CAD build for the part. Positions are in the model's coordinates, mm. Give positions to 0.01 mm unless a question says otherwise; leave off trailing zeros. Order: outer loops, then holes, each group sorted by start corner. A loop starts at its lowest first (then second) coordinate and runs counter-clockwise, first axis right, second up.
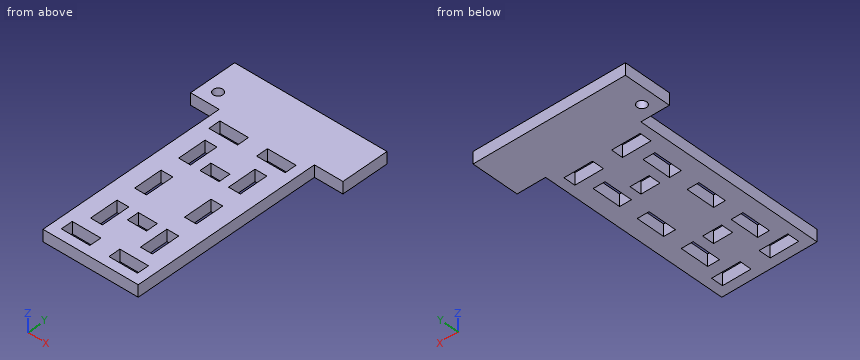
```python
from build123d import *

# Parameters (mm, degrees)
MODEL_R             = 5
MODEL_W             = 12.4
MODEL_H             = 30
MODEL_W_2           = 20
MODEL_H_2           = 12.4
MODEL_W_3           = 30
BOSS_EXTRUDE1_DEPTH = 12.4


with BuildPart() as part:
    # Model → Boss-Extrude1 (new body)
    with BuildSketch(Plane.XY):
        Polygon((50, 200), (80, 200), (80, 250), (-80, 250), (-80, 200), (-50, 200), (-50, 0), (50, 0), align=None)
        with Locations(Location((-65, 215, 0), (0, 0, 180))):
            Circle(MODEL_R, mode=Mode.SUBTRACT)
        with Locations((-26.2, 150)):
            Rectangle(MODEL_W, MODEL_H, mode=Mode.SUBTRACT)
        with Locations((-26.2, 100)):
            Rectangle(MODEL_W, MODEL_H, mode=Mode.SUBTRACT)
        with Locations((-26.2, 50)):
            Rectangle(MODEL_W, MODEL_H, mode=Mode.SUBTRACT)
        with Locations((26.2, 50)):
            Rectangle(MODEL_W, MODEL_H, mode=Mode.SUBTRACT)
        with Locations((26.2, 150)):
            Rectangle(MODEL_W, MODEL_H, mode=Mode.SUBTRACT)
        with Locations((26.2, 100)):
            Rectangle(MODEL_W, MODEL_H, mode=Mode.SUBTRACT)
        with Locations((0, 141.2)):
            Rectangle(MODEL_W_2, MODEL_H_2, mode=Mode.SUBTRACT)
        with Locations((0, 58.8)):
            Rectangle(MODEL_W_2, MODEL_H_2, mode=Mode.SUBTRACT)
        with Locations((25, 16.2)):
            Rectangle(MODEL_W_3, MODEL_H_2, mode=Mode.SUBTRACT)
        with Locations((-25, 16.2)):
            Rectangle(MODEL_W_3, MODEL_H_2, mode=Mode.SUBTRACT)
        with Locations((25, 183.8)):
            Rectangle(MODEL_W_3, MODEL_H_2, mode=Mode.SUBTRACT)
        with Locations((-25, 183.8)):
            Rectangle(MODEL_W_3, MODEL_H_2, mode=Mode.SUBTRACT)
    extrude(amount=BOSS_EXTRUDE1_DEPTH)


solid = part.part
```
Item 1: Wall check: L1, parallel to Y at x = -36, z = 10; L2, parallel to Y at x = -7.5, z = 3.5; L3, parallel to Y at x = 22.5, z = 6.5. Give the ranges that are in metal, low to high.
Item 2: Drop flat-ended pins along their axis: pin 1 Ø6 at (y, z) = (43, 3) entering from +X; pin 2 Ø6 at (y, z) = (45, 5.5) entering from -X; pin 3 Ø3.5 at (x, z) = (-30, 7) entering from -Y. Give the stop position or say it passes through.
Item 3: Slice it at A-A (y = 215). Give the cut face in (x, z).
Item 4: Slice it at C-C (y = 47). Give the cut face in (x, z), and give its area (3 significant figures).
Item 5: Slice it at D-D (x = -65). Give the cut face in (y, z), and give its area (3 significant figures).
Item 6: Slice it at B-B (x = -7). Give the cut face in (y, z), and give its area (3 significant figures).
A:
1. L1: y = 0 to 10, 22.4 to 177.6, 190 to 250
1. L2: y = 0 to 52.6, 65 to 135, 147.4 to 250
1. L3: y = 0 to 10, 22.4 to 35, 65 to 85, 115 to 135, 165 to 177.6, 190 to 250
2. pin 1: stops at x = 50
2. pin 2: stops at x = -50
2. pin 3: stops at y = 0
3. outline: (-80, 0) - (-70, 0) - (-70, 12.4) - (-80, 12.4) - close; (-60, 0) - (80, 0) - (80, 12.4) - (-60, 12.4) - close
4. outline: (-50, 0) - (-32.4, 0) - (-32.4, 12.4) - (-50, 12.4) - close; (-20, 0) - (20, 0) - (20, 12.4) - (-20, 12.4) - close; (32.4, 0) - (50, 0) - (50, 12.4) - (32.4, 12.4) - close
4. area: 932 mm2
5. outline: (200, 0) - (210, 0) - (210, 12.4) - (200, 12.4) - close; (220, 0) - (250, 0) - (250, 12.4) - (220, 12.4) - close
5. area: 496 mm2
6. outline: (0, 0) - (52.6, 0) - (52.6, 12.4) - (0, 12.4) - close; (65, 0) - (135, 0) - (135, 12.4) - (65, 12.4) - close; (147.4, 0) - (250, 0) - (250, 12.4) - (147.4, 12.4) - close
6. area: 2,790 mm2
